Can you work these out from the drawing? Everything is in mm from the part's minimum corner. A direction names the side the tool comes from. Coordinates: 2 decimals unless noted, no trailing zeros. Order: outer loops, then holes, each group sorted by start corner. A loop starts at its lowest first (then second) coordinate and runs counter-clockwise, first axis right, second up. Notation, with made-up numbers: (76, 8.25) - (98, 8.25) arc R33 ccw to (98, 47.25) - close; hole circle Ø5 at (28, 13). An arc over 180 degrees is marked (long way). Use a Markdown table: item, result. Add a question column.
(1) I want a section at B-B (x = 50). List the corners of the cut face in (y, z) for me.
(2) I want a section at A-A (y = 55). List the corners of the cut face in (x, z) for me.
(3) On a 3-axis mill with a long thin cutter (end or side, diameter ignored), from which of +Z, -Z, +X, -X, +Y, -Y can I reach the whole of each face in a straight line? I mean the marked faces 1 and 2. Say none if no direction works.
(4) If I drill on L1, parallel to X at y = 12, z = 15; L2, parallel to Y at x = 76.5, z = 26.5; L3, parallel to Y at x = 10.75, z = 15, over which ranges is the centre line in solid material (lowest first)? Write a range as [from, to].
(5) I want a section at D-D (y = 13.5). List the corners of the cut face in (x, z) for me, and give its area (3 significant figures).
(6) We'd pull the mould along X, two halves only. Please class the marked faces 3, 4 and 5: pulls with the +X half, pulls with the -X half, needs draft (parallel to the pull), parting line crosses it, or undercut.
(7) I want a section at C-C (z = 15). List the corners of the cut face in (x, y) for me.
(8) For pin 1 Ø6 at (x, y) = (48.5, 11.5) entering from -Z; pin 2 Ø1.5 at (y, z) = (29, 18) entering from +X; pin 3 Ø2 at (x, z) = (56.5, 26.5) entering from +Y; pin 4 Ø6 at (y, z) = (55, 15) entering from -X, each with a flat end and sliding along its axis, tell me the tip position at first contact or that it passes through.
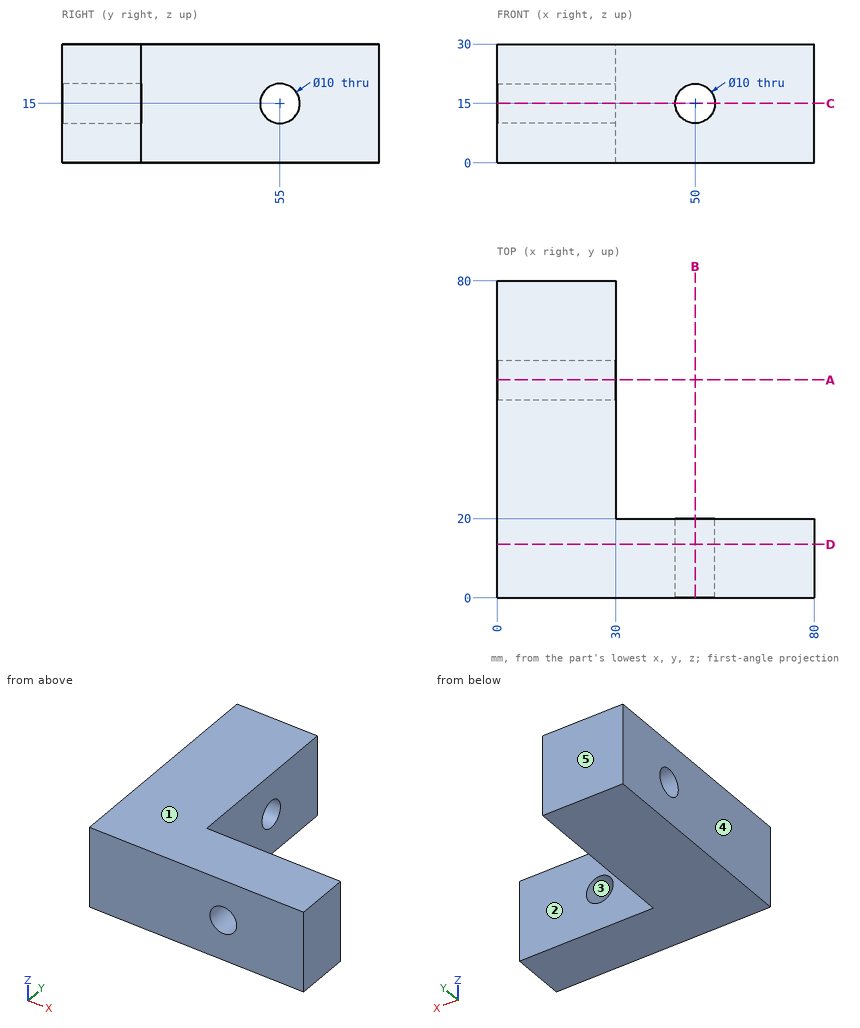
Answers follow:
| question | item | result |
|---|---|---|
| 1 | outline | (0, 0) - (20, 0) - (20, 10) - (0, 10) - close; (0, 20) - (20, 20) - (20, 30) - (0, 30) - close |
| 2 | outline | (0, 0) - (30, 0) - (30, 10) - (0, 10) - close; (0, 20) - (30, 20) - (30, 30) - (0, 30) - close |
| 3 | face 1 | +Z, +X, -X, +Y, -Y |
| 3 | face 2 | +Z, -Z, +X, +Y |
| 4 | L1 | x = [0, 45], [55, 80] |
| 4 | L2 | y = [0, 20] |
| 4 | L3 | y = [0, 50], [60, 80] |
| 5 | outline | (0, 0) - (80, 0) - (80, 30) - (0, 30) - close; hole circle Ø10 at (50, 15) |
| 5 | area | 2,320 mm² |
| 6 | face 3 | undercut |
| 6 | face 4 | pulls with the -X half |
| 6 | face 5 | needs draft |
| 7 | outline | (0, 0) - (45, 0) - (45, 20) - (30, 20) - (30, 50) - (0, 50) - close; (0, 60) - (30, 60) - (30, 80) - (0, 80) - close; (55, 0) - (80, 0) - (80, 20) - (55, 20) - close |
| 8 | pin 1 | stops at z = 0 |
| 8 | pin 2 | stops at x = 30 |
| 8 | pin 3 | stops at y = 20 |
| 8 | pin 4 | passes through |
